Read the model definition and answer for the solid it produces. Units are mm, in the model's axes. A direction names the side the tool comes from. Round coordinates to 2 decimals unless told otherwise and drop trailing zeros. Order: outer loops, then holes, each group sorted by start corner. A loop starts at its lowest first (then second) coordinate and runs counter-clockwise, first axis right, second up. Notation, with made-up numbers: M -24.75,-18.5 L 17.25,-18.5 A27 ccw 17.25,9.5 Z; hole C 18.5,20.5 d1. An arc over 180 degrees is marked long. Use one line per item in the form item = value. Start each with the question number.
Autodesk Inventor part; units mm, degrees
ref_plane "YZ Plane" through (0, 0, 0) normal (1, 0, 0) x (0, 1, 0)
ref_plane "XZ Plane" through (0, 0, 0) normal (0, 1, 0) x (-1, 0, 0)
ref_plane "XY Plane" through (0, 0, 0) normal (0, 0, 1) x (1, 0, 0)
sketch "Boceto1" plane through (0, 0, 0) normal (0, 1, 0) x (-1, 0, 0)
  line L0 (0, -10) -> (44.14, -10)
  line L1 (44.14, -10) -> (44.14, 0)
  line L2 (44.14, 0) -> (4.14, 0)
  line L3 (4.14, 0) -> (14.14, 0) construction
  line L4 (4.14, 0) -> (14.14, 0) construction
  line L5 (-5.86, 10) -> (4.14, 0)
  line L6 (-10, 0) -> (0, -10)
  line L7 (-10, 0) -> (-45.86, 0)
  line L8 (-10, 0) -> (25.86, 0) construction
  line L9 (-45.86, 0) -> (-45.86, 10)
  line L10 (-45.86, 10) -> (-5.86, 10)
  point P0 (0, 0)
  dimension "d10" = 44.14
  dimension "d12" = 40
  dimension "d19" = 35.86
  dimension "d21" = 10
extrude "Extrusión1" add sketch "Boceto1" along normal blind 30
sketch "Boceto2" plane through (5.86, 0, 10) normal (0, 0, 1) x (1, 0, 0)
  point P0 (-5.86, 0)
sketch "Boceto3" plane through (0, 0, -10) normal (0, 0, -1) x (-1, 0, 0)
  line L0 (44.14, 0) -> (44.14, 30)
  line L1 (0, 0) -> (0, 30)
  line L2 (44.14, 0) -> (44.14, 15)
  line L3 (44.14, 0) -> (59.14, 0) construction
  circle A0 centre (29.14, 15) radius 10
  line L4 (0, 0) -> (44.14, 0)
  line L5 (29.14, 15) -> (44.14, 15) construction
  arc A1 (29.14, 0) -> (29.14, 30) centre (29.14, 15) ccw
  line L6 (44.14, 30) -> (29.14, 30)
  line L7 (44.14, 0) -> (29.14, 0)
  dimension "d24" = 44.14
  dimension "d26" = 90
  dimension "d29" = 15
  dimension "d30" = 15
extrude "Extrusión2" cut sketch "Boceto3" against normal blind 30
sketch "Boceto4" plane through (5.86, 0, 10) normal (0, 0, 1) x (1, 0, 0)
  line L0 (40, 30) -> (4.14, 30)
  line L1 (40, 30) -> (40, 15)
  line L2 (40, 0) -> (40, 30)
  circle A0 centre (25, 15) radius 7.5
  circle A1 centre (25, 15) radius 10
  arc A2 (25, 0) -> (25, 30) centre (25, 15) ccw
  line L3 (40, 0) -> (25, 0)
  point P0 (-5.86, 0)
  dimension "d34" = 15
  dimension "d37" = 15
extrude "Extrusión3" cut sketch "Boceto4" against normal blind 30 contours L1 A2 L0 | L2 L3 A2
sketch "Boceto5" plane through (5.86, 0, 10) normal (0, 0, 1) x (1, 0, 0)
  arc A0 (25, 0) -> (25, 30) centre (25, 15) ccw
  line L0 (40, 15) -> (25, 15)
  circle A1 centre (25, 15) radius 10
  point P0 (-5.86, 0)
  dimension "d41" = 20
extrude "Extrusión4" add sketch "Boceto5" along normal blind 20
sketch "Boceto6" plane through (30.86, 15, 30) normal (0, 0, 1) x (1, 0, 0)
  line L0 (-25, 15) -> (0, 15)
  arc A0 (0, -15.2696) -> (0, 15) centre (-0.1195, -0.1348) ccw
  line L1 (0, 15) -> (0, -15.2696)
extrude "Extrusión5" add sketch "Boceto6" along normal blind 10
sketch "Boceto7" plane through (0, 30, 0) normal (0, 1, 0) x (1, 0, 0)
  line L0 (20.86, -30) -> (30.86, -30)
  line L1 (30.86, -30) -> (5.86, -30)
  line L2 (30.86, -30) -> (30.86, -40)
  line L3 (30.86, -40) -> (10, -40)
  line L4 (0, -50) -> (10, -40)
  line L5 (-4.14, -30) -> (5.86, -30) construction
  line L6 (-4.14, -40) -> (5.86, -30)
  line L7 (-4.14, -40) -> (-44.14, -40)
  line L8 (-4.14, -40) -> (35.86, -40) construction
  line L9 (-44.14, -40) -> (-44.14, -50)
  line L10 (-44.14, -50) -> (0, -50)
  point P0 (0, 0)
  dimension "d46" = 25
  dimension "d51" = 10
  dimension "d53" = 40
  dimension "d54" = 180
  dimension "d55" = 10
  dimension "d56" = 90
extrude "Extrusión6" add sketch "Boceto7" against normal blind 30
sketch "Boceto8" plane through (-44.14, 30, 50) normal (0, 0, 1) x (1, 0, 0)
  line L0 (40, 0) -> (0, 0)
  circle A0 centre (15, -15) radius 10
  circle A1 centre (15, -15) radius 10
  line L1 (0, 0) -> (0, -30)
  arc A2 (15, 0) -> (14.9869, -30) centre (14.9869, -15) ccw
  line L2 (0, -30) -> (40, -30)
  line L3 (14.9869, -30) -> (0, -30)
  point P0 (44.14, -30)
  point P1 (0, -14.3743)
  point P2 (0, -15.6257)
  dimension "d61" = 20
extrude "Extrusión7" cut sketch "Boceto8" against normal blind 30 contours A2 L1 L0 | A2 L2 L1 | A0
sketch "Boceto9" plane through (30.86, 15, 40) normal (0, 0, 1) x (1, 0, 0)
  circle A0 centre (0, 0) radius 7.5
  point P0 (-30.86, -15)
  dimension "d65" = 15
extrude "Extrusión8" cut sketch "Boceto9" against normal blind 60
Item 1: Section B-B (z = 46.5) is taken. Write down the section's boundary in (x, y), and give its area (3 significant figures).
Item 2: Find the intervals of material crossed by L1, parallel to Y at x = 30.86, z = 20.5; L2, parallel to Z at x = -40, y = 21; L3, parallel to Z at x = 23.5, y = 6, in increasing order. Write a range as [from, to].
Item 3: Given P1, Ø9, axis at x = 32.5, y = 20.5, coming from the -Z side; P2, Ø12, axis at x = 30.86, y = 15, coming from the +Z side; P3, Ø12, axis at x = -29.5, y = 20, coming from the +Z side; P4, Ø3, axis at x = 18.5, y = 19.5, coming from the +Z side, each flat-ended and moving along its own axis, determine where each tip first touches the part or whether it passes through.
Item 4: A tool of negligible diameter and unlimited length cuts with its end or side. For faces 1 (the flat face through (20, 15, 40)), 2 (the flat face through (0, 0, 40)), 3 (the flat face through (-19, 19, 40)), 4 (the flat face through (21, 12, 30)), from which of +Z, -Z, +X, -X, +Y, -Y can it reach the whole face along a straight path? Write none if from no direction.
Item 5: Section D-D (y = 2.5) is taken. Write down the section's boundary in (x, z).
Item 6: For a pull along Y with two mould halves and no side action, classify faces 5 (the cylindrical face through (38, 17.3, 20.3)), 6 (the flat face through (-16, 15, 0)), 7 (the cylindrical face through (45.856, 14.67, 5.07)) as pulls with the +Y half, pulls with the -Y half, needs draft (parallel to the pull), parting line crosses it, or undercut.
Item 7: Section A-A (x = 27) is taken. Write down the section's boundary in (y, z).
Item 8: Section C-C (y = 11.5) is taken. Give the number of separate pieces and of enclosed holes in the cut face, and give its area (3 significant figures).
The answers:
q1.outline = M -44.14,14.37 A15 ccw -29.15,0 L 3.5,0 L 3.5,30 L -29.14,30 A15 ccw -44.14,15.63 Z; hole C -29.14,15 d20
q1.area = 1,020 mm²
q2.L1 = [5, 7.5], [22.5, 25]
q2.L2 = [-10, 0], [40, 50]
q2.L3 = [0, 10], [30, 40]
q3.P1 = 0
q3.P2 = through
q3.P3 = 50
q3.P4 = 40
q4.face_1 = +Z, +X, +Y, -Y
q4.face_2 = +Z, -Z, -X, -Y
q4.face_3 = -X, +Y, -Y
q4.face_4 = none
q5.outline = M -37.44,40 L -4.14,40 L 5.86,30 L 39.47,30 L 39.47,40 L 10,40 L 0,50 L -37.44,50 Z; M -37.43,-10 L 0,-10 L 10,0 L 39.15,0 L 39.15,10 L 5.86,10 L -4.14,0 L -37.43,0 Z
q6.face_5 = undercut
q6.face_6 = needs draft
q6.face_7 = parting line crosses it
q7.outline = M 0,0 L 8.57,0 L 8.57,40 L 0,40 L 0,30 L 5.78,30 L 5.78,10 L 0,10 Z; M 21.43,0 L 30,0 L 30,10 L 24.22,10 L 24.22,30 L 30,30 L 30,40 L 21.43,40 Z
q8.separate_pieces = 4
q8.enclosed_holes = 0
q8.area = 1,340 mm²
